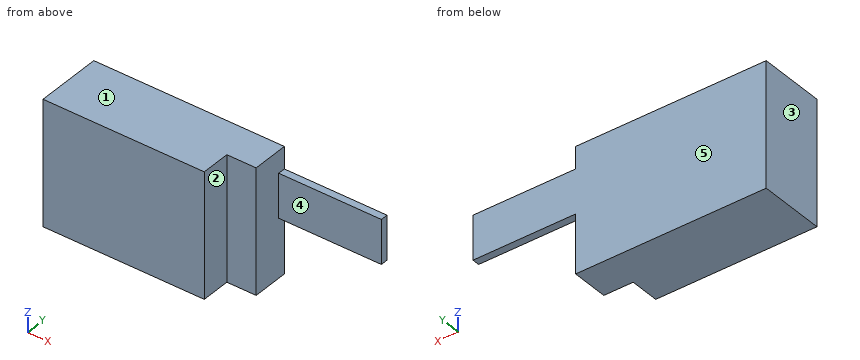
```python
from build123d import *

# Parameters (mm, degrees)
SKETCH1_W           = 82.55
SKETCH1_H           = 53.975
BOSS_EXTRUDE1_DEPTH = 28.575
SKETCH2_W           = 12.7
SKETCH2_H           = 12.7
CUT_EXTRUDE1_DEPTH  = 54.975
SKETCH3_W           = 44.45
SKETCH3_H           = 19.05
BOSS_EXTRUDE2_DEPTH = 3.175


with BuildPart() as part:
    # Sketch1 → Boss-Extrude1 (new body)
    with BuildSketch(Plane(origin=(0, 0, 0), x_dir=(1, 0, 0), z_dir=(0, 1, 0))):
        Rectangle(SKETCH1_W, SKETCH1_H)
    extrude(amount=BOSS_EXTRUDE1_DEPTH)

    # Sketch2 → Cut-Extrude1 (cut, through all)
    with BuildSketch(Plane.XY.offset(26.9875)):
        with Locations((34.925, 6.35)):
            Rectangle(SKETCH2_W, SKETCH2_H)
    extrude(amount=-CUT_EXTRUDE1_DEPTH, mode=Mode.SUBTRACT)

    # Sketch3 → Boss-Extrude2 (add)
    with BuildSketch(Plane(origin=(0, 28.575, 0), x_dir=(1, 0, 0), z_dir=(0, 1, 0))):
        with Locations((63.5, -7.9375)):
            Rectangle(SKETCH3_W, SKETCH3_H)
    extrude(amount=-BOSS_EXTRUDE2_DEPTH)


solid = part.part
```
For this review, take the finished solid that the model builds, in its own axes (mm). Face numbers are marked on the shaded views. A direction names the side the tool comes from. Give positions to 0.01 mm unless a question says otherwise; leave off trailing zeros. Write each loop counter-clockwise with the first axis right and the second up, starting at its lowest first coordinate (ties: lowest second). Pieces come first, ordered by that corner, then holes.
Item 1: Insertion check: P1, Ø8, axis at y = 21, z = 3, coming from the +X side (3 decimals); P2, Ø2.5, axis at x = 73.5, y = 27.5, coming from the +Z side; P3, Ø15, axis at x = 60.5, z = 11, coming from the -Y side. Each pin has a flat end and moves straight along its axis. Give the tip position at first contact, or say it passes through.
Item 2: Take a section at C-C (y = 10.25). Give the boundary of the cut face in (x, z) (1 decimal).
Item 3: Take a section at B-B (x = 58). Give the boundary of the cut face in (y, z) (1 decimal).
Item 4: The part is to be moulded in two halves that separate along X. For the marked faces 1, 2 and 3, say which applies: +X half, -X half, draft (parallel to the pull), parting line (faces both ways), or undercut.
Item 5: Machinability: for the marked faces 4 and 5, which of the approach directions +Z, -Z, +X, -X, +Y, -Y give a long, thin tool a straight path to every point of the face, cutting with its end or side? Answer none if there is none.
Item 6: Take a section at D-D (z = 10.5). Give the boundary of the cut face in (x, y) (3 decimals).
Item 7: Wall thickness on probe 1 along X at (y, z) = (16.25, 22.5) (3 decimals); probe 2 along Y at (x, z) = (31, 7.5) (3 decimals); probe 3 along Y at (x, z) = (56, 17) (3 decimals): over which ranges is each line inside the solid? List them lowest first.
Item 8: Take a section at A-A (z = -7). Give the boundary of the cut face in (x, y) (3 decimals), and give its area (3 significant figures).
Established:
1. P1: stops at x = 41.275
1. P2: stops at z = 17.46
1. P3: stops at y = 25.4
2. outline: (-41.3, -27) - (28.6, -27) - (28.6, 27) - (-41.3, 27) - close
3. outline: (25.4, -1.6) - (28.6, -1.6) - (28.6, 17.5) - (25.4, 17.5) - close
4. face 1: draft
4. face 2: +X half
4. face 3: -X half
5. face 4: +Z, -Z, +X, -Y
5. face 5: +Z, -Z, +X, -X, +Y
6. outline: (-41.275, 0) - (28.575, 0) - (28.575, 12.7) - (41.275, 12.7) - (41.275, 25.4) - (85.725, 25.4) - (85.725, 28.575) - (-41.275, 28.575) - close
7. probe 1: x = -41.275 to 41.275
7. probe 2: y = 12.7 to 28.575
7. probe 3: y = 25.4 to 28.575
8. outline: (-41.275, 0) - (28.575, 0) - (28.575, 12.7) - (41.275, 12.7) - (41.275, 28.575) - (-41.275, 28.575) - close
8. area: 2,200 mm2
